Verification items for the finished model (mm, model axes). A direction names the side the tool comes from. Round coordinates to 2 decimals unless told otherwise and drop trailing zeros. Write each loop counter-clockwise with the first axis right and the second up, starting at its lowest first coordinate (ties: lowest second). Pieces come first, ordered by that corner, then holes. Notation, with made-up numbers: M 49.5,12 L 102.5,12 A28 ccw 102.5,34 Z; hole C 3,11 d2. An arc over 180 degrees is marked long. One line per item, written item: value. Start each with the question number.
from build123d import *

# Parameters (mm, degrees)
F0_W     = 29.938724
F0_H     = 30
F1_DEPTH = 36
F2_T     = -2.41
F3_SIZE  = 0.1


with BuildPart() as f1:
    # F0 (on Front) → F1 (new body)
    with BuildSketch(Plane.XZ):
        with Locations((14.969362, 15)):
            Rectangle(F0_W, F0_H)
    extrude(amount=F1_DEPTH)

    # F2
    f2_openings = [f1.faces().sort_by_distance(p)[0] for p in [
        (14.969362, -36, 15),
    ]]
    offset(amount=F2_T, openings=f2_openings)

    # F3
    f3_edges = [f1.edges().sort_by_distance(p)[0] for p in [
        (29.938724, 0, 15),
    ]]
    chamfer(f3_edges, length=F3_SIZE)


solid = f1.part
1) Cross-section at C-C (x = 24.5). Record the boundary of the cut face in (y, z).
2) Mould release check, pull along X, two halves, no side actions. Record for faces 1 (the flat face through (2.41, -19, 15)), 2 (the flat face through (29.939, -18, 15)), 3 (the flat face through (15, 0, 15)): pulls with the +X half, pulls with the -X half, needs draft (parallel to the pull), parting line crosses it, or undercut.
3) Gauge pin test, flat end, axial feed: pin 1 Ø6 at (x, z) = (20.5, 6.5) entering from -Y. Record the tip position at first contact, or that the pin passes through.
4) Access from +Z, -Z, +X, -X, +Y, -Y to the whole of each face (thin tool, end or side, straight path). Record for faces 4 (the flat face through (15, -18, 0)), 5 (the flat face through (15, -19, 2.41)).
5) Cross-section at A-A (z = 24.5). Record the boundary of the cut face in (x, y).
6) Thickness scan on line 1 (X direction, y = -17.5, z = 20.5); line 2 (Z direction, x = 10.75, y = -4); line 3 (Y direction, x = 4.25, z = 18.25). Record the ranges inside material, lowest first.
7) Cross-section at B-B (y = -34). Record the boundary of the cut face in (x, z).
Results below:
1. outline: M -36,0 L 0,0 L 0,30 L -36,30 L -36,27.59 L -2.41,27.59 L -2.41,2.41 L -36,2.41 Z
2. face 1: undercut
2. face 2: pulls with the +X half
2. face 3: needs draft
3. pin 1: stops at y = -2.41
4. face 4: -Z, +X, -X, +Y, -Y
4. face 5: -Y
5. outline: M 0,-36 L 2.41,-36 L 2.41,-2.41 L 27.53,-2.41 L 27.53,-36 L 29.94,-36 L 29.94,-0.1 L 29.84,0 L 0,0 Z
6. line 1: x = 0 to 2.41, 27.53 to 29.94
6. line 2: z = 0 to 2.41, 27.59 to 30
6. line 3: y = -2.41 to 0
7. outline: M 0,0 L 29.94,0 L 29.94,30 L 0,30 Z; hole M 2.41,2.41 L 27.53,2.41 L 27.53,27.59 L 2.41,27.59 Z
